Check sheet for the drawn part. Datum: minimum x, y, z corner. Units: mm. Give positions to 0.01 mm unless a question says otherwise; leave off trailing zeros. Write each loop counter-clockwise with the first axis right and the second up, starting at its lowest first coordinate (ties: lowest second). Pieces come first, ordered by that corner, then holes. Notation, with made-up numbers: (54, -27.75) - (93, -27.75) arc R18 cw to (93, -4.75) - close; hole circle Ø3 at (57.25, 15.25). An arc over 180 degrees is marked (long way). One line per question, with ' | ' between items. Start each with the question number.
Q1. Release check for a two-part mould opening along Z. For the marked faces 1, 2 and 3 record: +Z half, -Z half, draft (parallel to the pull), parting line (faces both ways), or undercut.
Q2. Section check B-B on x = 41.2. Record the boundary of the cut face in (y, z).
Q3. Section check A-A on z = 45.95. Record the boundary of the cut face in (x, y), and give its area (3 significant figures).
Q4. Thickness scan on L1, parallel to Y at x = 45.95, z = 88.85; L2, parallel to Z at x = 41, y = 1 (1 decimal); L3, parallel to Y at x = 45, z = 88. Record the ranges inside material, lowest first. Write a range as [from, to].
Q5. Section check C-C on y = 7. Record the boundary of the cut face in (x, z), and give its area (4 significant figures).
Q6. Gauge pin test, flat ends, axial feed: P1, Ø2.5, axis at x = 41.2, z = 54.18, coming from the +Y side; P2, Ø10, axis at x = 14, y = 28.5, coming from the -Z side; P3, Ø2, axis at x = 50.7, z = 54.18, coming from the +Y side; P4, Ø3, axis at y = 29.5, z = 48.5, coming from the -X side. Record the tip position at first contact, or that the pin passes through.
Q7. Section check D-D on z = 57. Record the boundary of the cut face in (x, y).
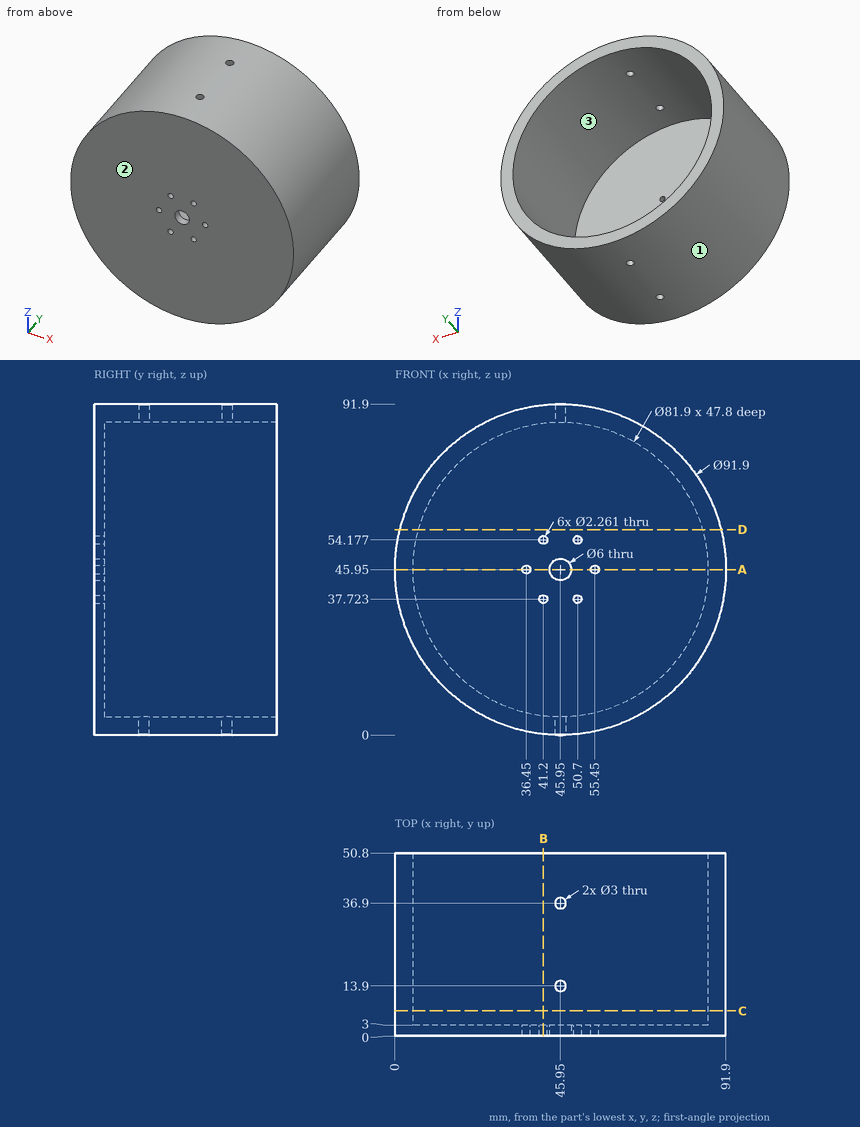
Working result:
1) face 1: parting line | face 2: draft | face 3: undercut
2) outline: (0, 0.25) - (50.8, 0.25) - (50.8, 5.28) - (3, 5.28) - (3, 36.59) - (0, 36.59) - close; (0, 38.85) - (3, 38.85) - (3, 53.05) - (0, 53.05) - close; (0, 55.31) - (3, 55.31) - (3, 86.62) - (50.8, 86.62) - (50.8, 91.65) - (0, 91.65) - close
3) outline: (0, 0) - (35.32, 0) - (35.32, 3) - (5, 3) - (5, 50.8) - (0, 50.8) - close; (37.58, 0) - (42.95, 0) - (42.95, 3) - (37.58, 3) - close; (48.95, 0) - (54.32, 0) - (54.32, 3) - (48.95, 3) - close; (56.58, 0) - (91.9, 0) - (91.9, 50.8) - (86.9, 50.8) - (86.9, 3) - (56.58, 3) - close | area: 722 mm2
4) L1: y = [0, 12.4], [15.4, 35.4], [38.4, 50.8] | L2: z = [0.3, 36.6], [38.8, 53.1], [55.3, 91.6] | L3: y = [0, 12.74], [15.06, 35.74], [38.06, 50.8]
5) outline: circle Ø91.9 at (45.95, 45.95); hole circle Ø81.9 at (45.95, 45.95) | area: 1,365 mm2
6) P1: stops at y = 3 | P2: stops at z = 8.73 | P3: passes through | P4: stops at x = 0.01
7) outline: (1.35, 0) - (90.55, 0) - (90.55, 50.8) - (85.38, 50.8) - (85.38, 3) - (6.52, 3) - (6.52, 50.8) - (1.35, 50.8) - close
